Build history of the part. All positions in model axes, mm. Give positions to 0.01 mm unless a question says otherwise; leave off trailing zeros. Order: outer loops, then holes, each group sorted by start corner. A loop starts at its lowest first (then second) coordinate and runs counter-clockwise, first axis right, second up. Notation, with made-up numbers: (67, -4) - (101, -4) arc R26 ccw to (101, 20) - close; hole circle Ø3 at (-0.75, 50.5). An arc over 180 degrees is marked (long way). Use a Markdown table: item, result.
from build123d import *

# Parameters (mm, degrees)
SKETCH1_W                    = 3.175
SKETCH1_H                    = 12.7
MAIN_EXTRUDE_DEPTH           = 3.175
SKETCH8_R                    = 1.5
SKETCH8_W                    = 3.175
SKETCH8_H                    = 31.877
MOUNT_HOLES_DEPTH            = 4.175
DOOR_SLOTS_DEPTH             = 4.175
SKETCH4_W                    = 30.099999998
SKETCH4_H                    = 6.858
TROUGH_AND_LEVER_HOLES_DEPTH = 4.175
SKETCH10_R                   = 1.5
DOOR_GUIDE_MOUNT_HOLES_DEPTH = 4.175
SKETCH12_R                   = 1.5
EXTENSION_CLIP_HOLES_DEPTH   = 4.175
EXTENSION_CENTER_CUT_DEPTH   = 4.175


with BuildPart() as part:
    # Sketch1 → Main Extrude (new body)
    with BuildSketch(Plane.XY):
        Polygon((-243.84, -134.112), (-189.653333333, -134.112), (-189.653333333, -139.7), (-135.466666667, -139.7), (-135.466666667, -134.112), (-81.28, -134.112), (-81.28, -139.7), (-27.093333333, -139.7), (-27.093333333, -134.112), (27.093333333, -134.112), (27.093333333, -139.7), (81.28, -139.7), (81.28, -134.112), (135.466666667, -134.112), (135.466666667, -139.7), (189.653333333, -139.7), (189.653333333, -134.112), (243.84, -134.112), (243.84, -139.7), (298.026666667, -139.7), (298.026666667, -134.112), (352.213333333, -134.112), (352.213333333, -139.7), (406.4, -139.7), (406.4, 139.7), (381, 139.7), (381, 127), (377.825, 127), (377.825, 139.7), (-377.825, 139.7), (-377.825, 127), (-381, 127), (-381, 139.7), (-406.4, 139.7), (-406.4, -139.7), (-352.213333333, -139.7), (-352.213333333, -134.112), (-298.026666667, -134.112), (-298.026666667, -139.7), (-243.84, -139.7), align=None)
        with Locations((-379.4125, -120.65)):
            Rectangle(SKETCH1_W, SKETCH1_H, mode=Mode.SUBTRACT)
        with Locations((-379.4125, -95.25)):
            Rectangle(SKETCH1_W, SKETCH1_H, mode=Mode.SUBTRACT)
        with Locations((379.4125, 82.55)):
            Rectangle(SKETCH1_W, SKETCH1_H, mode=Mode.SUBTRACT)
        with Locations((379.4125, 57.15)):
            Rectangle(SKETCH1_W, SKETCH1_H, mode=Mode.SUBTRACT)
        with Locations((379.4125, 31.75)):
            Rectangle(SKETCH1_W, SKETCH1_H, mode=Mode.SUBTRACT)
        with Locations((379.4125, 6.35)):
            Rectangle(SKETCH1_W, SKETCH1_H, mode=Mode.SUBTRACT)
        with Locations((379.4125, -19.05)):
            Rectangle(SKETCH1_W, SKETCH1_H, mode=Mode.SUBTRACT)
        with Locations((379.4125, -44.45)):
            Rectangle(SKETCH1_W, SKETCH1_H, mode=Mode.SUBTRACT)
        with Locations((379.4125, -69.85)):
            Rectangle(SKETCH1_W, SKETCH1_H, mode=Mode.SUBTRACT)
        with Locations((379.4125, -95.25)):
            Rectangle(SKETCH1_W, SKETCH1_H, mode=Mode.SUBTRACT)
        with Locations((379.4125, -120.65)):
            Rectangle(SKETCH1_W, SKETCH1_H, mode=Mode.SUBTRACT)
        with Locations((-379.4125, -69.85)):
            Rectangle(SKETCH1_W, SKETCH1_H, mode=Mode.SUBTRACT)
        with Locations((-379.4125, -44.45)):
            Rectangle(SKETCH1_W, SKETCH1_H, mode=Mode.SUBTRACT)
        with Locations((-379.4125, -19.05)):
            Rectangle(SKETCH1_W, SKETCH1_H, mode=Mode.SUBTRACT)
        with Locations((-379.4125, 6.35)):
            Rectangle(SKETCH1_W, SKETCH1_H, mode=Mode.SUBTRACT)
        with Locations((-379.4125, 31.75)):
            Rectangle(SKETCH1_W, SKETCH1_H, mode=Mode.SUBTRACT)
        with Locations((-379.4125, 57.15)):
            Rectangle(SKETCH1_W, SKETCH1_H, mode=Mode.SUBTRACT)
        with Locations((-379.4125, 82.55)):
            Rectangle(SKETCH1_W, SKETCH1_H, mode=Mode.SUBTRACT)
        with Locations((-379.4125, 107.95)):
            Rectangle(SKETCH1_W, SKETCH1_H, mode=Mode.SUBTRACT)
        with Locations((379.4125, 107.95)):
            Rectangle(SKETCH1_W, SKETCH1_H, mode=Mode.SUBTRACT)
    extrude(amount=MAIN_EXTRUDE_DEPTH)

    # Sketch8 → Mount Holes (cut, through all)
    with BuildSketch(Plane.XY.offset(3.175)):
        with Locations((-393.7, -120.65)):
            Circle(SKETCH8_R)
        with Locations((393.7, -120.65)):
            Circle(SKETCH8_R)
        with Locations((-382.5875, 12.319)):
            Rectangle(SKETCH8_W, SKETCH8_H)
        with Locations((382.5875, 12.319)):
            Rectangle(SKETCH8_W, SKETCH8_H)
    extrude(amount=-MOUNT_HOLES_DEPTH, mode=Mode.SUBTRACT)

    # Sketch3 → Door Slots (cut, through all)
    with BuildSketch(Plane.XY.offset(3.175)):
        Polygon((-88.7095, 126.492), (-92.6465, 126.492), (-92.6465, 82.042), (-96.52, 82.042), (-96.52, 10.3505), (-106.553, 10.3505), (-106.553, 0.8255), (-96.52, 0.8255), (-96.52, -134.112), (-84.836, -134.112), (-84.836, 0.8255), (-74.803, 0.8255), (-74.803, 10.3505), (-84.836, 10.3505), (-84.836, 82.042), (-88.7095, 82.042), align=None)
        Polygon((92.6465, 126.492), (88.7095, 126.492), (88.7095, 82.042), (84.836, 82.042), (84.836, 10.3505), (74.803, 10.3505), (74.803, 0.8255), (84.836, 0.8255), (84.836, -134.112), (96.52, -134.112), (96.52, 0.8255), (106.553, 0.8255), (106.553, 10.3505), (96.52, 10.3505), (96.52, 82.042), (92.6465, 82.042), align=None)
    extrude(amount=-DOOR_SLOTS_DEPTH, mode=Mode.SUBTRACT)

    # Sketch4 → Trough and Lever Holes (cut, through all)
    with BuildSketch(Plane.XY):
        Polygon((-52.178, -134.112), (-52.178, -139.7), (-2.178, -139.7), (-2.178, -134.112), (1.124, -134.112), (1.124, -112.41), (-2.178, -112.41), (-2.178, -106.172), (-52.178, -106.172), (-52.178, -112.41), (-55.48, -112.41), (-55.48, -134.112), align=None)
        with Locations((27.178, -115.062)):
            Rectangle(SKETCH4_W, SKETCH4_H)
    extrude(amount=TROUGH_AND_LEVER_HOLES_DEPTH, mode=Mode.SUBTRACT)

    # Sketch10 → Door Guide Mount Holes (cut, through all)
    with BuildSketch(Plane.XY.offset(3.175)):
        with Locations((-101.678, 127.492)):
            Circle(SKETCH10_R)
        with Locations((-79.678, 127.492)):
            Circle(SKETCH10_R)
        with Locations((79.678, 127.492)):
            Circle(SKETCH10_R)
        with Locations((101.678, 127.492)):
            Circle(SKETCH10_R)
    extrude(amount=-DOOR_GUIDE_MOUNT_HOLES_DEPTH, mode=Mode.SUBTRACT)

    # Sketch12 → Extension Clip Holes (cut, through all)
    with BuildSketch(Plane.XY.offset(3.175)):
        with Locations((-246.507, 20.193)):
            Circle(SKETCH12_R)
        with Locations((-246.507, 4.445)):
            Circle(SKETCH12_R)
        with Locations((-221.107, 4.445)):
            Circle(SKETCH12_R)
        with Locations((-221.107, 20.193)):
            Circle(SKETCH12_R)
        with Locations((-243.332, 133.35)):
            Circle(SKETCH12_R)
        with Locations((-224.282, 133.35)):
            Circle(SKETCH12_R)
        with Locations((224.282, 133.35)):
            Circle(SKETCH12_R)
        with Locations((243.332, 133.35)):
            Circle(SKETCH12_R)
        with Locations((221.107, 20.193)):
            Circle(SKETCH12_R)
        with Locations((221.107, 4.445)):
            Circle(SKETCH12_R)
        with Locations((246.507, 4.445)):
            Circle(SKETCH12_R)
        with Locations((246.507, 20.193)):
            Circle(SKETCH12_R)
    extrude(amount=-EXTENSION_CLIP_HOLES_DEPTH, mode=Mode.SUBTRACT)

    # Sketch11_3 → Extension Center Cut (cut, through all)
    with BuildSketch(Plane.XY.offset(3.175)):
        Polygon((-232.2195, 127), (-232.2195, 139.7), (-406.4, 139.7), (-406.4, -139.7), (-235.3945, -139.7), (-235.3945, -127), (-232.2195, -127), (-232.2195, -114.3), (-235.3945, -114.3), (-235.3945, -101.6), (-232.2195, -101.6), (-232.2195, -88.9), (-235.3945, -88.9), (-235.3945, -76.2), (-232.2195, -76.2), (-232.2195, -63.5), (-235.3945, -63.5), (-235.3945, -50.8), (-232.2195, -50.8), (-232.2195, -38.1), (-235.3945, -38.1), (-235.3945, -25.4), (-232.2195, -25.4), (-232.2195, -12.7), (-235.3945, -12.7), (-235.3945, 0), (-232.2195, 0), (-232.2195, 12.7), (-235.3945, 12.7), (-235.3945, 25.4), (-232.2195, 25.4), (-232.2195, 38.1), (-235.3945, 38.1), (-235.3945, 50.8), (-232.2195, 50.8), (-232.2195, 63.5), (-235.3945, 63.5), (-235.3945, 76.2), (-232.2195, 76.2), (-232.2195, 88.9), (-235.3945, 88.9), (-235.3945, 101.6), (-232.2195, 101.6), (-232.2195, 114.3), (-235.3945, 114.3), (-235.3945, 127), align=None)
        Polygon((406.4, 139.7), (232.2195, 139.7), (232.2195, 127), (235.3945, 127), (235.3945, 114.3), (232.2195, 114.3), (232.2195, 101.6), (235.3945, 101.6), (235.3945, 88.9), (232.2195, 88.9), (232.2195, 76.2), (235.3945, 76.2), (235.3945, 63.5), (232.2195, 63.5), (232.2195, 50.8), (235.3945, 50.8), (235.3945, 38.1), (232.2195, 38.1), (232.2195, 25.4), (235.3945, 25.4), (235.3945, 12.7), (232.2195, 12.7), (232.2195, 0), (235.3945, 0), (235.3945, -12.7), (232.2195, -12.7), (232.2195, -25.4), (235.3945, -25.4), (235.3945, -38.1), (232.2195, -38.1), (232.2195, -50.8), (235.3945, -50.8), (235.3945, -63.5), (232.2195, -63.5), (232.2195, -76.2), (235.3945, -76.2), (235.3945, -88.9), (232.2195, -88.9), (232.2195, -101.6), (235.3945, -101.6), (235.3945, -114.3), (232.2195, -114.3), (232.2195, -127), (235.3945, -127), (235.3945, -139.7), (406.4, -139.7), align=None)
    extrude(amount=-EXTENSION_CENTER_CUT_DEPTH, mode=Mode.SUBTRACT)


solid = part.part
1) Slice it at C-C (z = 1.8). State how many separate pieces and enclosed holes the cut face has, and give its area (3 significant figures).
Computed:
| item | result |
|---|---|
| separate pieces | 1 |
| enclosed holes | 11 |
| area | 121,000 mm² |
2) Slice it at A-A (y = -20). Write the cut outline in (x, z) (1 decimal), and give its area (3 significant figures).
Computed:
| item | result |
|---|---|
| outline | (-232.2, 0) - (-96.5, 0) - (-96.5, 3.2) - (-232.2, 3.2) - close; (-84.8, 0) - (84.8, 0) - (84.8, 3.2) - (-84.8, 3.2) - close; (96.5, 0) - (232.2, 0) - (232.2, 3.2) - (96.5, 3.2) - close |
| area | 1,400 mm² |
3) Slice it at B-B (x = -38). Write the cut outline in (y, z) (3 decimals).
Computed:
| item | result |
|---|---|
| outline | (-106.172, 0) - (139.7, 0) - (139.7, 3.175) - (-106.172, 3.175) - close |
4) Pin check, flat tips, straight feed: P1, Ø1.6, axis at x = -233.5, z = 1.5, coming from the +Y side; P2, Ø2.5, axis at x = -79.678, y = 127.492, coming from the -Z side; P3, Ø1, axis at y = -72.5, z = 1.5, coming from the -X side; P4, Ø1.6, axis at x = 234.5, z = 1, coming from the -Y side. Stop position of each tip, or through.
Computed:
| item | result |
|---|---|
| P1 | stops at y = 127 |
| P2 | passes through |
| P3 | stops at x = -232.22 |
| P4 | stops at y = -134.11 |
5) Wall check: line 1 (X direction, y = 28, z = 2.95); line 2 (Y direction, x = 102, z = 0.45); line 3 (X direction, y = 1, z = 2.35). Give the ranges that are in metal, low to high. Write a range as from..to.
Computed:
| item | result |
|---|---|
| line 1 | x = -232.22..-96.52, -84.84..84.84, 96.52..232.22 |
| line 2 | y = -134.11..0.83, 10.35..126.03, 128.96..139.7 |
| line 3 | x = -232.22..-106.55, -74.8..74.8, 106.55..232.22 |
